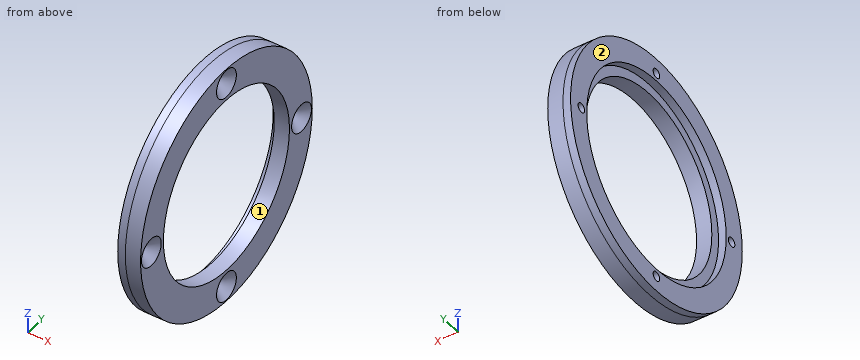
Solid Edge part; units mm, degrees
sketch "Sketch1" plane through (0, 0, 0) normal (1, 0, 0) x (0, 1, 0)
  circle A0 centre (0, 0) radius 16
  circle A1 centre (0, 0) radius 11.75
extrude "Protrusion1" add sketch "Sketch1" along normal blind 2
sketch "Sketch2" plane through (0, 0, 0) normal (-1, 0, 0) x (0, -1, 0)
  circle A0 centre (0, 0) radius 16
  circle A1 centre (0, 0) radius 13
extrude "Extrusionsausprägung_2" add sketch "Sketch2" along normal blind 1
hole "Bohrung_1" at (2, 14, 0) direction (-1, 0, 0) diameter 1.221 end up to next countersink diameter 3.7 countersink angle 90 thread major 1.6 thread length 2
pattern_circular "Pattern2" count 4 over 360 about axis through (2, 0, 0) along (1, 0, 0) of "Bohrung_1"
Source: CAD feature listing. Evaluate the final solid. Frame: model axes, mm. Face numbers are marked on the shaded views. Give positions to 0.01 mm unless a question says otherwise; leave off trailing zeros. Loops run counter-clockwise (first coordinate to the right, second up) from the corner with the lowest first, then second, coordinate; pieces in that order, holes last. Notation, with made-up numbers: (41, 22.5) -> (87, 22.5) arc R35 ccw to (87, 54.5) -> close; hole circle Ø11 at (-23.5, 57.25). An arc over 180 degrees is marked (long way). Use a Markdown table: item, result. Add a question column.
1) Section query C-C, the plane z = 3. Return the cut outline in (x, y).
2) Section query A-A, the plane z = 11. Return the cut outline in (x, y).
3) First-contact query: pin 1 (1.5 mm diameter, centred on x = 0.5, z = -8.5, fed in from -Y); pin 2 (1.5 mm diameter, centred on x = 0, y = 2, fed in from -Z); pin 3 (0.7 mm diameter, centred on y = -14, z = 0, fed in from +X); pin 4 (2 mm diameter, centred on y = 14, z = 0, fed in from +X). Flat tips, straight axial feed; report the tip coordinate or a pass-through.
4) Pull-direction query (Z, two-part tool) for the marked faces 1 and 2; classes: +Z half, -Z half, draft (parallel to the pull), parting line (faces both ways), or undercut.
5) Section query B-B, the plane y = -14. Return the cut outline in (x, z).
6) Line query: line 1 along Z through (x, y) = (0.4, 0); line 2 along Z through (x, y) = (-0.25, 0); line 3 along Z through (x, y) = (1.3, -4). Output: solid intervals per line, ascending. Write a range as [from, to].
Numbers:
| question | item | result |
|---|---|---|
| 1 | outline | (-1, -15.72) -> (2, -15.72) -> (2, -11.36) -> (0, -11.36) -> (0, -12.65) -> (-1, -12.65) -> close; (-1, 12.65) -> (0, 12.65) -> (0, 11.36) -> (2, 11.36) -> (2, 15.72) -> (-1, 15.72) -> close |
| 2 | outline | (-1, -11.62) -> (2, -11.62) -> (2, -4.13) -> (0, -4.13) -> (0, -6.93) -> (-1, -6.93) -> close; (-1, 6.93) -> (0, 6.93) -> (0, 4.13) -> (2, 4.13) -> (2, 11.62) -> (-1, 11.62) -> close |
| 3 | pin 1 | stops at y = -14 |
| 3 | pin 2 | stops at z = -15.95 |
| 3 | pin 3 | passes through |
| 3 | pin 4 | stops at x = 1.15 |
| 4 | face 1 | undercut |
| 4 | face 2 | draft |
| 5 | outline | (-1, -7.75) -> (2, -7.75) -> (2, -1.85) -> (0.76, -0.61) -> (-1, -0.61) -> close; (-1, 0.61) -> (0.76, 0.61) -> (2, 1.85) -> (2, 7.75) -> (-1, 7.75) -> close |
| 6 | line 1 | z = [-16, -14.61], [-13.39, -11.75], [11.75, 13.39], [14.61, 16] |
| 6 | line 2 | z = [-16, -14.61], [-13.39, -13], [13, 13.39], [14.61, 16] |
| 6 | line 3 | z = [-15.49, -11.05], [11.05, 15.49] |
